```python
from build123d import *

# Parameters (mm, degrees)
F0_W     = 32.5
F0_H     = 20
F1_DEPTH = 88
F2_T     = -2
F4_DEPTH = 25


with BuildPart() as f1:
    # F0 (on Front) → F1 (new body)
    with BuildSketch(Plane.XZ):
        with Locations((16.25, -10)):
            Rectangle(F0_W, F0_H)
    extrude(amount=F1_DEPTH)

    # F2
    f2_openings = [f1.faces().sort_by_distance(p)[0] for p in [
        (16.25, -44, 0),
    ]]
    offset(amount=F2_T, openings=f2_openings)

    # F3 (on face) → F4 (cut)
    with BuildSketch(Plane.XZ.offset(88)):
        with BuildLine():
            Line((23.75, -2.428177), (8.75, -2.428177))
            ThreePointArc((8.75, -2.428177), (6.25, -4.928177), (8.75, -7.428177))
            Line((8.75, -7.428177), (23.75, -7.428177))
            ThreePointArc((23.75, -7.428177), (26.25, -4.928177), (23.75, -2.428177))
        make_face()
    extrude(amount=-F4_DEPTH, mode=Mode.SUBTRACT)


solid = f1.part
```
Design review of the part built by this model. Coordinates are the model's own, in mm. A direction names the side the tool comes from. Coordinates: 2 decimals unless noted, no trailing zeros. Order: outer loops, then holes, each group sorted by start corner. A loop starts at its lowest first (then second) coordinate and runs counter-clockwise, first axis right, second up. Notation, with made-up numbers: M -12,3.5 L 25,3.5 A13 ccw 25,27.5 Z; hole C 8.5,77.5 d2. An arc over 180 degrees is marked long. Answer as a JSON object with one key per item and string values. Group by question number.
1) Mouldability with a two-part tool opening along Y and no side actions: class faces 4 (the flat face through (16, -2, -9)), 5 (the flat face through (16, -88, -10)), 6 (the flat face through (1.7, -40.5, 0)), 7 (the flat face through (2, -43, -9)) as pulls with the +Y half, pulls with the -Y half, needs draft (parallel to the pull), parting line crosses it, or undercut.
2) Tool access review of faces 1 (the flat face through (32.5, -43, -10)), 2 (the flat face through (16, -87, -7.428)), 3 (the flat face through (30.5, -43, -9)): name each direction out of +Z, -Z, +X, -X, +Y, -Y from which nothing blocks a thin tool from reaching the whole face with its end or side.
3) Add section C-C, the plane y = -34. Write out the cut boundary in (x, z), then the cut area to 3 significant figures.
4) Add section A-A, the plane x = 22.5. Write out the cut boundary in (y, z).
5) Add section D-D, the plane x = 3.5. Write out the cut boundary in (y, z).
6) For pin 1 (12 mm diameter, centred on x = 13.5, y = -56, fed in from +Z), flat-tipped, find the tip position at first contact; note if it passes through.
7) Add section B-B, the plane z = -16. Write out the cut boundary in (x, y).
8) Wall thickness on L1, parallel to X at y = -55, z = -12.5; L2, parallel to Y at x = 10, z = -11.25; L3, parallel to Z at x = 3.5, y = -65.5: over which ranges is each line inside the solid? List them lowest first.
Computed values:
{
 "1": {"face 4": "undercut", "face 5": "pulls with the -Y half", "face 6": "needs draft", "face 7": "undercut"},
 "2": {"face 1": "+Z, -Z, +X, +Y, -Y", "face 2": "-Y", "face 3": "+Z"},
 "3": {"outline": "M 0,-20 L 32.5,-20 L 32.5,0 L 30.5,0 L 30.5,-18 L 2,-18 L 2,0 L 0,0 Z", "area": "137 mm^2"},
 "4": {"outline": "M -88,-20 L 0,-20 L 0,0 L -2,0 L -2,-18 L -86,-18 L -86,-7.43 L -88,-7.43 Z; M -88,-2.43 L -86,-2.43 L -86,0 L -88,0 Z"},
 "5": {"outline": "M -88,-20 L 0,-20 L 0,0 L -2,0 L -2,-18 L -86,-18 L -86,0 L -88,0 Z"},
 "6": {"pin 1": "stops at z = -18"},
 "7": {"outline": "M 0,-88 L 32.5,-88 L 32.5,0 L 0,0 Z; hole M 2,-86 L 30.5,-86 L 30.5,-2 L 2,-2 Z"},
 "8": {"L1": "x = 0 to 2, 30.5 to 32.5", "L2": "y = -88 to -86, -2 to 0", "L3": "z = -20 to -18"}
}
